```python
from build123d import *

# Parameters (mm, degrees)
F2_R = 0.508
F3_R = 0.508


with BuildPart() as f1:
    # F0 (on Front) → F1 (revolve)
    with BuildSketch(Plane.XZ):
        Polygon((5.9055, 10.234522), (5.9055, 17.854522), (2.3495, 17.854522), (2.3495, -7.545478), (5.9055, -7.545478), (5.9055, 0.074522), (3.6195, 0.074522), (3.6195, 10.234522), align=None)
    revolve(axis=Axis((0, 0, 1.306427), (0, 0, 1)))

    # F2
    f2_edges = [f1.edges().sort_by_distance(p)[0] for p in [
        (-5.9055, 0, 17.854522),
        (-5.9055, 0, 10.234522),
        (-5.9055, 0, 0.074522),
    ]]
    fillet(f2_edges, radius=F2_R)

    # F3
    f3_edges = [f1.edges().sort_by_distance(p)[0] for p in [
        (-5.9055, 0, -7.545478),
    ]]
    fillet(f3_edges, radius=F3_R)


solid = f1.part
```
Geometry: final body of the model. Coordinates: model frame, mm. A direction names the side the tool comes from. Coordinates: 2 decimals unless noted, no trailing zeros. Loops run counter-clockwise (first coordinate to the right, second up) from the corner with the lowest first, then second, coordinate; pieces in that order, holes last. Notation, with made-up numbers: M 81.25,-5.5 L 130.25,-5.5 A25 cw 130.25,17.5 Z; hole C 81,33 d5. An arc over 180 degrees is marked long. Put each result on its own line as item: value.
(1) Access query for faces 1 (the face through (-4.69, -3.59, -3.69)), 2 (the face through (1, -4, 0.075)). Directions: +Z, -Z, +X, -X, +Y, -Y. A direction counts if a zero-diameter tool reaches every point of the face in a straight line with its end or side. Return the directions, or none.
Answer sheet:
face 1: +Z, -Z
face 2: none
(2) Cut plane D-D on z = 15. Return the cut outline in (x, y).
Answer sheet:
outline: C 0,0 d11.81; hole C 0,0 d4.7
(3) Cut plane A-A on x = 0. Return the cut outline in (y, z), then the cut area to 3 significant figures.
Answer sheet:
outline: M -5.91,-7.04 A0.51 ccw -5.4,-7.55 L -2.35,-7.55 L -2.35,17.85 L -5.4,17.85 A0.51 ccw -5.91,17.35 L -5.91,10.74 A0.51 ccw -5.4,10.23 L -3.62,10.23 L -3.62,0.07 L -5.4,0.07 A0.51 ccw -5.91,-0.43 Z; M 2.35,-7.55 L 5.4,-7.55 A0.51 ccw 5.91,-7.04 L 5.91,-0.43 A0.51 ccw 5.4,0.07 L 3.62,0.07 L 3.62,10.23 L 5.4,10.23 A0.51 ccw 5.91,10.74 L 5.91,17.35 A0.51 ccw 5.4,17.85 L 2.35,17.85 Z
area: 134 mm^2
(4) Material intervals for probe 1 along Z at (x, y) = (3.25, -2); probe 2 along Y at (x, z) = (0, 10); probe 3 along Z at (x, y) = (-2, -5.25), sorted ascending.
Answer sheet:
probe 1: z = -7.55 to 0.07, 10.23 to 17.85
probe 2: y = -3.62 to -2.35, 2.35 to 3.62
probe 3: z = -7.5 to 0.02, 10.28 to 17.8
(5) First-contact query: pin 1 (1.5 mm diameter, centred on x = 1.5, z = 12, fed in from +Y); pin 2 (2 mm diameter, centred on y = 4, z = -2.5, fed in from -X). Flat tips, straight axial feed; report the tip coordinate or a pass-through.
Answer sheet:
pin 1: stops at y = 5.86
pin 2: stops at x = -5.09
(6) Cut plane C-C on z = 3.5. Return the cut outline in (x, y), then the cut area to 3 significant figures.
Answer sheet:
outline: C 0,0 d7.24; hole C 0,0 d4.7
area: 23.8 mm^2
(7) Draft query along Z for faces 3 (the face through (-4.69, -3.59, 14.09)), 4 (the face through (-0.47, 3.59, 5.23)), 5 (the face through (-1.1, -2.3, -7.545)). Return one class per face: pulls with the +Z half, pulls with the -Z half, needs draft (parallel to the pull), parting line crosses it, or undercut.
Answer sheet:
face 3: needs draft
face 4: undercut
face 5: pulls with the -Z half
